Input: dimensioned drawing with shaded views. Units: mm. Origin: part minimum x, y, z. A direction names the side the tool comes from. Round coordinates to 2 decimals unless told otherwise and drop trailing zeros. Loops run counter-clockwise (first coordinate to the right, second up) from the corner with the lowest first, then second, coordinate; pieces in that order, holes last. Notation, with made-up numbers: M 38,19.5 L 54,19.5 A18 cw 54,26.5 Z; hole C 60,67 d1. An arc over 180 degrees is marked long. Answer as CSV lines item,"result". Start each with the question number.
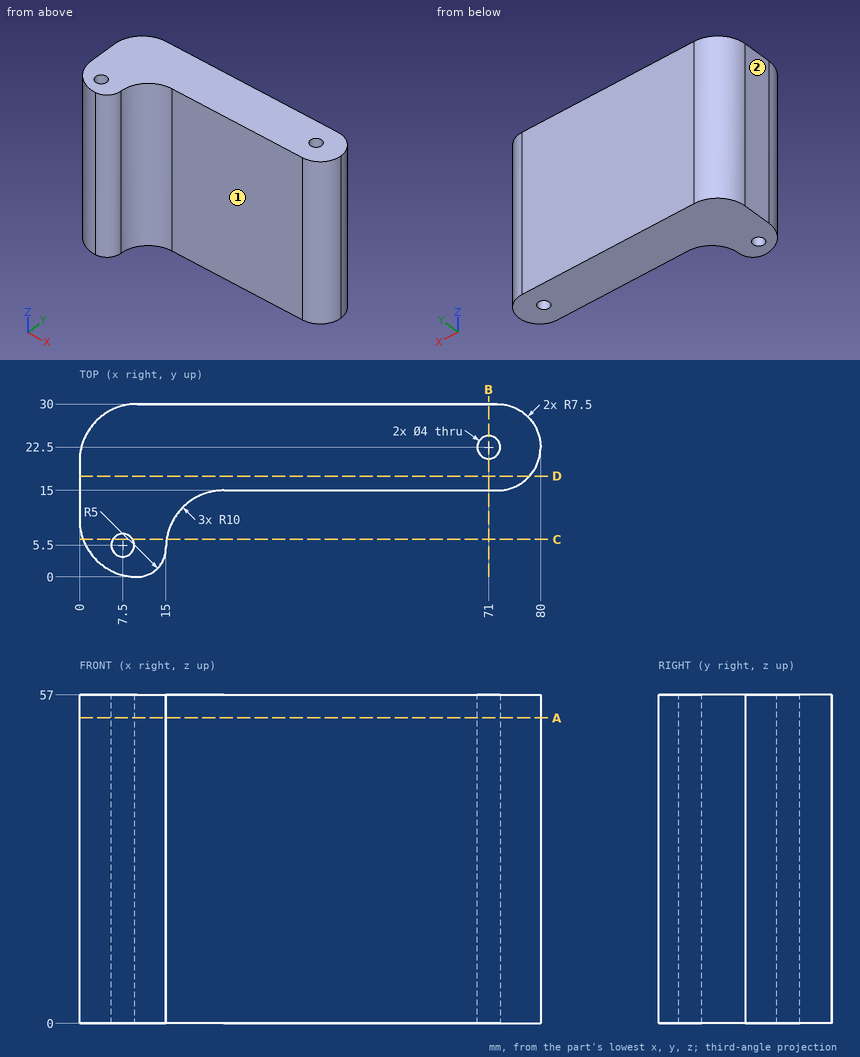
1) Ray query, line 1 along Y through (x, z) = (71, 41); line 2 along X through (y, z) = (3.75, 10.5) (1 decimal); line 3 along Y through (x, z) = (28, 37.5). Return the intervals inside material, ascending.
2) Access query for the marked faces 1 and 2. Directions: +Z, -Z, +X, -X, +Y, -Y. A direction counts if a zero-diameter tool reaches every point of the face in a straight line with its end or side. Return the directions, or none.
3) Section C-C, the plane y = 6.5. Return loops of the section in (x, z), and give its area (3 significant figures).
4) Section D-D, the plane y = 17.5. Return loops of the section in (x, z).
5) Section B-B, the plane x = 71. Return loops of the section in (y, z).
6) Section A-A, the plane z = 53. Give the number of separate pieces and of enclosed holes in the cut face, and give its area (3 significant figures).
7) Contact query for flat-ended pins moving along their axis: pin 1 Ø2 at (x, z) = (34.5, 43) entering from -Y; pin 2 Ø12 at (x, z) = (30, 49.5) entering from -Y; pin 3 Ø1 at (y, z) = (20.5, 7.5) entering from +X. Output: stop coordinate, or through.
Findings below:
1,line 1,"15 to 20.5, 24.5 to 30"
1,line 2,"2.2 to 6.5, 8.5 to 14.8"
1,line 3,"15 to 30"
2,face 1,"+Z, -Z, +X, -Y"
2,face 2,"+Z, -Z, -X, +Y, -Y"
3,outline,"M 0.63,0 L 5.77,0 L 5.77,57 L 0.63,57 Z; M 9.23,0 L 15.11,0 L 15.11,57 L 9.23,57 Z"
3,area,"628 mm²"
4,outline,"M 0,0 L 78.09,0 L 78.09,57 L 0,57 Z"
5,outline,"M 15,0 L 20.5,0 L 20.5,57 L 15,57 Z; M 24.5,0 L 30,0 L 30,57 L 24.5,57 Z"
6,separate pieces,"1"
6,enclosed holes,"2"
6,area,"1,350 mm²"
7,pin 1,"y = 15"
7,pin 2,"y = 14.95"
7,pin 3,"x = 79.85"
